Study the drawing (mm; zero at the part's minimum x, y, z) and answer. A direction names the side the tool comes from. Give positions to 0.01 mm unless a question says otherwise; leave off trailing zeros. Order: outer loops, then holes, each group sorted by start corner. A loop starts at its lowest first (then second) coordinate and runs counter-clockwise, first axis right, second up. Notation, with made-up numbers: (47.5, 60) -> (101.5, 60) arc R11 cw to (101.5, 73) -> close; hole circle Ø7 at (77, 48). An arc over 180 degrees is marked (long way). Use a Markdown table: item, result. Add a question column.
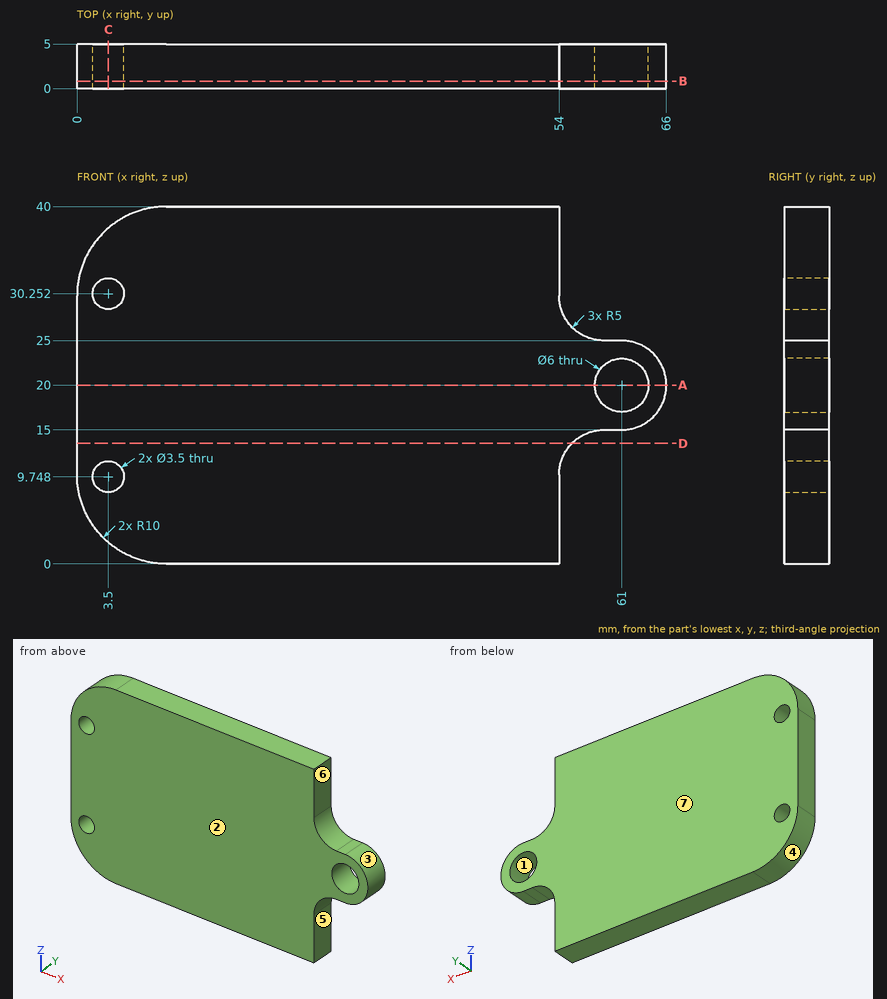
1) Flat-ended cylindrical pins translate along their axes: pin 1 (2 mm diameter, centred on x = 60, y = 2.5, fed in from -Z); pin 2 (1 mm diameter, centred on x = 60, y = 1.5, fed in from +Z). Find the tip coordinate at first contact, or state that the pin passes through.
2) Determine the mould class of the marked faces 1, 2, 3 and 4 for opening direction X: released by +X, released by -X, zero draft, split by the parting line, or undercut.
3) Which of the six approach directions +Z, -Z, +X, -X, +Y, -Y give full straight-line access (tool end or side, diameter ignored) to the marked faces 5, 6 and 7?
4) The part is cut by section A-A, the plane z = 20. Determine the outline of the cut face in (x, y), then the cut area to 3 significant figures.
5) Straight lines are drawn through the part: line 1 (X direction, y = 0.3, z = 30); line 2 (X direction, y = 1.95, z = 12.5); line 3 (X direction, y = 1.6, z = 8.5). For each, find the intervals that lie inside material, in ascending order.
6) The part is cut by section C-C, the plane x = 3.5. Determine the outline of the cut face in (y, z).
7) The part is cut by section B-B, the plane y = 0.85. Determine the outline of the cut face in (x, z), then the cut area to 3 significant figures.
8) The part is cut by section D-D, the plane z = 13.5. Determine the outline of the cut face in (x, y), then the cut area to 3 significant figures.
A:
| question | item | result |
|---|---|---|
| 1 | pin 1 | z = 15 |
| 1 | pin 2 | z = 25 |
| 2 | face 1 | undercut |
| 2 | face 2 | zero draft |
| 2 | face 3 | released by +X |
| 2 | face 4 | released by -X |
| 3 | face 5 | -Z, +X, +Y, -Y |
| 3 | face 6 | +Z, +X, +Y, -Y |
| 3 | face 7 | +Z, -Z, +X, -X, +Y |
| 4 | outline | (0, 0) -> (58, 0) -> (58, 5) -> (0, 5) -> close; (64, 0) -> (66, 0) -> (66, 5) -> (64, 5) -> close |
| 4 | area | 300 mm^2 |
| 5 | line 1 | 0 to 1.77, 5.23 to 54 |
| 5 | line 2 | 0 to 54.67 |
| 5 | line 3 | 0.11 to 2.27, 4.73 to 54 |
| 6 | outline | (0, 2.4) -> (5, 2.4) -> (5, 8) -> (0, 8) -> close; (0, 11.5) -> (5, 11.5) -> (5, 28.5) -> (0, 28.5) -> close; (0, 32) -> (5, 32) -> (5, 37.6) -> (0, 37.6) -> close |
| 7 | outline | (0, 10) arc R10 ccw to (10, 0) -> (54, 0) -> (54, 10) arc R5 cw to (59, 15) -> (61, 15) arc R5 ccw to (61, 25) -> (59, 25) arc R5 cw to (54, 30) -> (54, 40) -> (10, 40) arc R10 ccw to (0, 30) -> close; hole circle Ø3.5 at (3.5, 9.75); hole circle Ø3.5 at (3.5, 30.25); hole circle Ø6 at (61, 20) |
| 7 | area | 2,190 mm^2 |
| 8 | outline | (0, 0) -> (55.43, 0) -> (55.43, 5) -> (0, 5) -> close |
| 8 | area | 277 mm^2 |
